Geometry check sheet. Reference: the model listing, model coordinates, mm. Face numbers are marked on the shaded views. A direction names the side the tool comes from. Coordinates: 2 decimals unless noted, no trailing zeros. Loops run counter-clockwise (first coordinate to the right, second up) from the corner with the lowest first, then second, coordinate; pieces in that order, holes last.
from build123d import *

# Parameters (mm, degrees)
F1_DEPTH = 85
F3_DEPTH = 2.801


with BuildPart() as f1:
    # F0 (on Front) → F1 (new body, symmetric)
    with BuildSketch(Plane.XZ):
        with BuildLine():
            Line((18.652306, 40), (3.714916, 7.966662))
            ThreePointArc((3.714916, 7.966662), (4.067247, 2.591122), (8.790239, 0))
            Line((8.790239, 0), (77.590239, 0))
            ThreePointArc((77.590239, 0), (82.31449, 2.593095), (82.663585, 7.970904))
            Line((82.663585, 7.970904), (67.726194, 40.004241))
            Line((67.726194, 40.004241), (65.188533, 38.82091))
            Line((65.188533, 38.82091), (80.127901, 6.783331))
            ThreePointArc((80.127901, 6.783331), (79.951735, 4.095561), (77.590239, 2.8))
            Line((77.590239, 2.8), (8.790239, 2.8))
            ThreePointArc((8.790239, 2.8), (6.428743, 4.095561), (6.252577, 6.783331))
            Line((6.252577, 6.783331), (21.189968, 38.816669))
            Line((21.189968, 38.816669), (18.652306, 40))
        make_face()
    extrude(amount=F1_DEPTH, both=True)

    # F2 (on face) → F3 (cut, through all)
    with BuildSketch(Plane.XY.offset(2.8)):
        with BuildLine():
            Line((49.190239, -85), (49.190239, -45))
            ThreePointArc((49.190239, -45), (43.190239, -39), (37.190239, -45))
            Line((37.190239, -45), (37.190239, -85))
            Line((37.190239, -85), (49.190239, -85))
        make_face()
        with BuildLine():
            Line((49.190239, 45), (49.190239, 85))
            Line((49.190239, 85), (37.190239, 85))
            Line((37.190239, 85), (37.190239, 45))
            ThreePointArc((37.190239, 45), (43.190239, 39), (49.190239, 45))
        make_face()
    extrude(amount=-F3_DEPTH, mode=Mode.SUBTRACT)


solid = f1.part
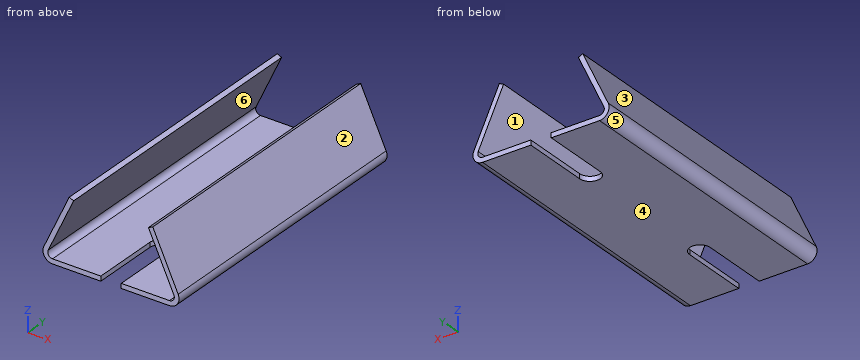
(1) Gauge pin test, flat ends, axial feed: pin 1 Ø1.5 at (y, z) = (-64, 20.5) entering from +X; pin 2 Ø0.8 at (y, z) = (-57.5, 1) entering from +X; pin 3 Ø3 at (x, y) = (19, 3.5) entering from +Z. Record the tip position at first contact, or that the pin passes through.
Findings:
pin 1: stops at x = 77.17
pin 2: stops at x = 81.29
pin 3: stops at z = 40
(2) Draft check along Z on the marked faces 3, 4, 5 and 6. Enter one of: +Z half, -Z half, draft (parallel to the pull), parting line (faces both ways), or undercut.
Findings:
face 3: +Z half
face 4: -Z half
face 5: parting line
face 6: undercut
(3) Sectioned sample at A-A on x = 75. Record the cut outline in (y, z), and give its area (3 significant figures).
Findings:
outline: (-85, 0) - (85, 0) - (85, 2.8) - (-85, 2.8) - close; (-85, 17.78) - (85, 17.78) - (85, 24.41) - (-85, 24.41) - close
area: 1,600 mm2
(4) Access from +Z, -Z, +X, -X, +Y, -Y to the whole of each face (thin tool, end or side, straight path). Record for the marked faces 1 and 2.
Findings:
face 1: +Y, -Y
face 2: +Z, +X, +Y, -Y
(5) Sectioned sample at D-D on x = 60. Record the cut outline in (y, z).
Findings:
outline: (-85, 0) - (85, 0) - (85, 2.8) - (-85, 2.8) - close
(6) Scan lines: L1, parallel to X at y = -52, z = 32; L2, parallel to Z at x = 42, y = 11; L3, parallel to X at y = -52.5, z = 18. Record each from-to range of solid material in increasing order.
Findings:
L1: x = 14.92 to 18.01, 68.37 to 71.46
L2: z = 0 to 2.8
L3: x = 8.39 to 11.48, 74.9 to 77.99
(7) Sectioned sample at C-C on z = 13.5. Record the cut outline in (x, y), and give its area (3 significant figures).
Findings:
outline: (6.3, -85) - (9.38, -85) - (9.38, 85) - (6.3, 85) - close; (77, -85) - (80.09, -85) - (80.09, 85) - (77, 85) - close
area: 1,050 mm2
(8) Sectioned sample at B-B on y = 22. Record the cut outline in (x, z), and give its area (3 significant figures).
Findings:
outline: (3.71, 7.97) arc R5.6 ccw to (8.79, 0) - (77.59, 0) arc R5.6 ccw to (82.66, 7.97) - (67.73, 40) - (65.19, 38.82) - (80.13, 6.78) arc R2.8 cw to (77.59, 2.8) - (8.79, 2.8) arc R2.8 cw to (6.25, 6.78) - (21.19, 38.82) - (18.65, 40) - close
area: 438 mm2
